Autodesk Inventor part; units mm, degrees
ref_plane "YZ Plane" through (0, 0, 0) normal (1, 0, 0) x (0, 1, 0)
ref_plane "XZ Plane" through (0, 0, 0) normal (0, 1, 0) x (-1, 0, 0)
ref_plane "XY Plane" through (0, 0, 0) normal (0, 0, 1) x (1, 0, 0)
sketch "Sketch1" plane through (0, 0, 0) normal (0, 0, 1) x (1, 0, 0)
  line L0 (0, 0) -> (6.35, 0)
  line L1 (6.35, 0) -> (6.35, 6.35)
  line L2 (6.35, 6.35) -> (0, 6.35)
  line L3 (0, 6.35) -> (0, 0)
  dimension "d0" = 6.35
  dimension "d1" = 6.35
extrude "Extrusion1" add sketch "Sketch1" along normal blind 6.35
sketch "Sketch2" plane through (6.35, 0, 0) normal (1, 0, 0) x (0, 0, -1)
  line L0 (0, 6.35) -> (-6.35, 6.35)
  line L1 (-4.7625, 6.35) -> (-1.5875, 6.35)
  line L2 (0, 0) -> (0, 6.35)
  line L3 (-6.35, 0) -> (-6.35, 6.35)
  line L4 (-6.35, 4.7625) -> (0, 4.7625)
  line L5 (0, 4.7625) -> (0, 1.5875)
  line L6 (0, 1.5875) -> (-6.35, 1.5875)
  line L7 (-6.35, 1.5875) -> (-6.35, 4.7625)
  line L8 (0, 0) -> (-6.35, 0)
  dimension "d13" = 3.175
  dimension "d14" = 1.5875
sketch "Sketch3" plane through (0, 0, 0) normal (0, -1, 0) x (1, 0, 0)
  line L0 (6.35, 0) -> (0, 0)
  line L1 (1.5875, 6.35) -> (4.7625, 6.35)
  line L2 (4.7625, 6.35) -> (4.7625, 0)
  line L3 (4.7625, 0) -> (1.5875, 0)
  line L4 (1.5875, 0) -> (1.5875, 6.35)
  line L5 (6.35, 0) -> (6.35, 6.35)
  line L6 (0, 6.35) -> (6.35, 6.35)
  line L7 (0, 0) -> (0, 6.35)
  point P0 (6.35, 4.7625)
  dimension "d9" = 3.175
  dimension "d10" = 0
  dimension "d17" = 1.5875
extrude "Extrusion3" add sketch "Sketch3" along normal blind 6.35 contours L0 L4 L1 L2
extrude "Extrusion4" add sketch "Sketch2" along normal blind 6.35 contours L2 L6 L3 L4
fillet "Fillet1" radius 3.175 1 edges at (0, 6.35, 3.175)
properties part number "MonsterHolderSupport3"
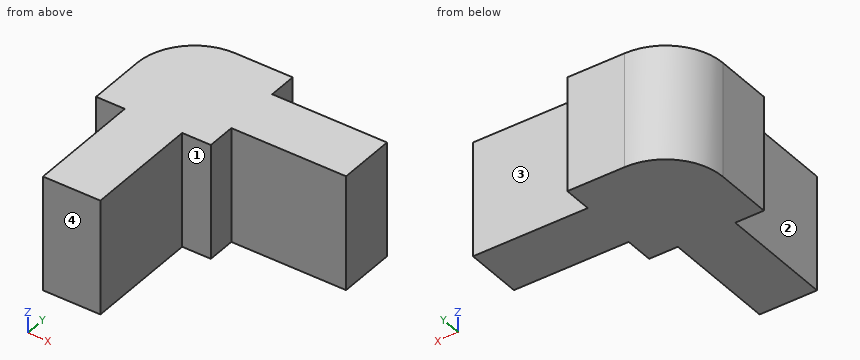
Here's how the part is built. I have some questions about the finished solid (model axes, mm). Face numbers are marked on the shaded views. A direction names the side the tool comes from. Give positions to 0.01 mm unless a question says otherwise; leave off trailing zeros. Order: outer loops, then holes, each group sorted by start corner. A loop starts at its lowest first (then second) coordinate and runs counter-clockwise, first axis right, second up. Notation, with made-up numbers: M 64,-31.5 L 83,-31.5 A20 ccw 83,-12.5 Z; hole C 43,27 d3. An arc over 180 degrees is marked long. Use a Markdown table: item, result. Add a question column.
1. I need wall thicknesses on probe 1 along X at (y, z) = (-4.75, 0.5); probe 2 along X at (y, z) = (3.25, 4.75); probe 3 along Y at (x, z) = (6, 4). Which ranges of each line are inside material? Lowest first, please. Write a range as from..to.
2. For pin 1 Ø3 at (x, z) = (9, 2.5) entering from +Y; pin 2 Ø3 at (y, z) = (-3, 1.5) entering from +X; pin 3 Ø0.5 at (x, z) = (1, 4.5) entering from -Y, each with a flat end and sliding along its axis, tell me the tip position at first contact or that it passes through.
3. Suppose I cut it at B-B (y = -3). List the corners of the cut face in (x, z) for me, and give its area (3 significant figures).
4. On a 3-axis mill with a long thin cutter (end or side, diameter ignored), from which of +Z, -Z, +X, -X, +Y, -Y can I reach the whole of each face in a straight line? I mean the marked faces 1, 2, 3 and 4. Say none if no direction works.
5. Suppose I cut it at C-C (x = 5). List the corners of the cut face in (y, z) for me.
Results list:
| question | item | result |
|---|---|---|
| 1 | probe 1 | x = 1.59..4.76 |
| 1 | probe 2 | x = 0..12.7 |
| 1 | probe 3 | y = 0..6.35 |
| 2 | pin 1 | stops at y = 4.76 |
| 2 | pin 2 | stops at x = 4.76 |
| 2 | pin 3 | stops at y = 0 |
| 3 | outline | M 1.59,0 L 4.76,0 L 4.76,6.35 L 1.59,6.35 Z |
| 3 | area | 20.2 mm² |
| 4 | face 1 | +Z, -Z, +X, -Y |
| 4 | face 2 | +Z, -Z, -X, -Y |
| 4 | face 3 | +Z, -Z, +X, +Y |
| 4 | face 4 | +Z, -Z, +X, -X, -Y |
| 5 | outline | M 0,0 L 6.35,0 L 6.35,6.35 L 0,6.35 Z |
